from build123d import *

# Parameters (mm, degrees)
F1_DEPTH = 6
F2_W     = 6
F2_H     = 5
F3_DEPTH = 3
F4_R     = 1
F5_DEPTH = 100


with BuildPart() as f1:
    # F0 (on Top) → F1 (new body)
    with BuildSketch(Plane.XY):
        Polygon((0, 3.382515), (-72, 40.882515), (-72, 34.117485), (-6.494428, 0), (-72, -34.117485), (-72, -40.882515), (0, -3.382515), (72, -40.882515), (72, -34.117485), (6.494428, 0), (72, 34.117485), (72, 40.882515), align=None)
    extrude(amount=F1_DEPTH)

    # F2 (on Top) → F3 (join)
    with BuildSketch(Plane.XY):
        with Locations((-75, 37.5)):
            Rectangle(F2_W, F2_H)
        with Locations((-75, -37.5)):
            Rectangle(F2_W, F2_H)
        with Locations((75, -37.5)):
            Rectangle(F2_W, F2_H)
        with Locations((75, 37.5)):
            Rectangle(F2_W, F2_H)
    extrude(amount=F3_DEPTH)

    # F4 (on face) → F5 (cut)
    with BuildSketch(Plane.XZ.offset(40)):
        with BuildLine():
            ThreePointArc((-76, 3), (-75, 2), (-74, 3))
            Line((-74, 3), (-76, 3))
        make_face()
        with Locations((75, 3)):
            Circle(F4_R)
    extrude(amount=-F5_DEPTH, mode=Mode.SUBTRACT)


solid = f1.part
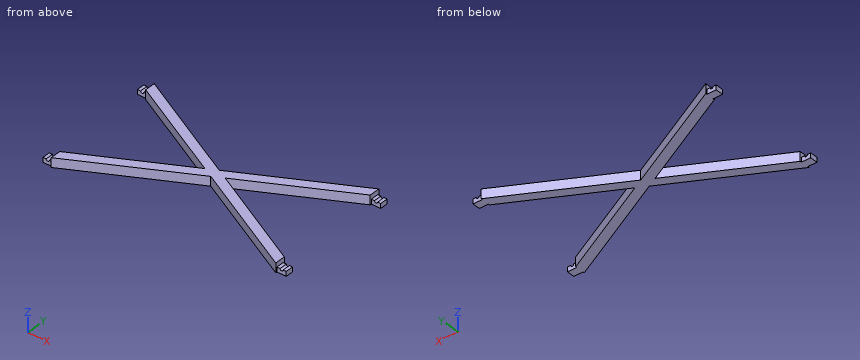
For this review, take the finished solid that the model builds, in its own axes (mm). Round coordinates to 2 decimals unless told otherwise and drop trailing zeros. Loops run counter-clockwise (first coordinate to the right, second up) from the corner with the lowest first, then second, coordinate; pieces in that order, holes last. Notation, with made-up numbers: (84, -36.5) - (130, -36.5) arc R36 cw to (130, 2.5) - close; hole circle Ø7 at (27, 13). An arc over 180 degrees is marked (long way). One line per question, with ' | ' between items.
Q1. For pin 1 (0.9 mm diameter, centred on x = -74.5, z = 2, fed in from -Y); pin 2 (1.5 mm diameter, centred on x = 2, z = 0.5, fed in from -Y); pin 3 (1 mm diameter, centred on x = 77, y = 38.5, fed in from +Z), all flat-tipped, find the tip position at first contact; note any pin that passes through.
Taken from the geometry:
pin 1: stops at y = -40 | pin 2: stops at y = -4.81 | pin 3: stops at z = 3
Q2. Take a section at B-B (x = -49.5). Give the boundary of the cut face in (y, z), and give its area (3 significant figures).
Taken from the geometry:
outline: (-29.16, 0) - (-22.4, 0) - (-22.4, 6) - (-29.16, 6) - close; (22.4, 0) - (29.16, 0) - (29.16, 6) - (22.4, 6) - close | area: 81.2 mm²
Q3. For line 1 along Y through (x, z) = (-14, 1.4); line 2 along Y through (x, z) = (-31, 3.3); line 3 along X through (y, z) = (32.5, 2.45), list the stretches that pass through material, from the lowest coordinate up. Write a range as [from, to].
Taken from the geometry:
line 1: y = [-10.67, -3.91], [3.91, 10.67] | line 2: y = [-19.53, -12.76], [12.76, 19.53] | line 3: x = [-68.89, -55.91], [55.91, 68.89]
Q4. Take a section at C-C (y = 18). Give the boundary of the cut face in (x, z), and give its area (3 significant figures).
Taken from the geometry:
outline: (-41.05, 0) - (-28.07, 0) - (-28.07, 6) - (-41.05, 6) - close; (28.07, 0) - (41.05, 0) - (41.05, 6) - (28.07, 6) - close | area: 156 mm²
Q5. Take a section at A-A (z = 4.7). Give the boundary of the cut face in (x, y), and give its area (3 significant figures).
Taken from the geometry:
outline: (-72, -40.88) - (0, -3.38) - (72, -40.88) - (72, -34.12) - (6.49, 0) - (72, 34.12) - (72, 40.88) - (0, 3.38) - (-72, 40.88) - (-72, 34.12) - (-6.49, 0) - (-72, -34.12) - close | area: 1,900 mm²
